from build123d import *

# Parameters (mm, degrees)
SKETCH1_R           = 6.22935
BOSS_EXTRUDE1_DEPTH = 31.75
SKETCH2_W           = 8.89
SKETCH2_H           = 31.75
CUT_EXTRUDE1_DEPTH  = 89.9


with BuildPart() as part:
    # Sketch1 → Boss-Extrude1 (new body)
    with BuildSketch(Plane(origin=(0, 0, 0), x_dir=(0, 0, -1), z_dir=(1, 0, 0))):
        with BuildLine():
            Line((22.594948, 7.845241626), (32.874076775, 30.623791868))
            ThreePointArc((32.874076775, 30.623791868), (44.45, 38.1), (56.025923225, 30.623791868))
            Line((56.025923225, 30.623791868), (66.305052, 7.845241626))
            ThreePointArc((66.305052, 7.845241626), (67.242210206, 6.756307629), (68.620236645, 6.35))
            Line((68.620236645, 6.35), (88.9, 6.35))
            Line((88.9, 6.35), (88.9, 0))
            Line((88.9, 0), (0, 0))
            Line((0, 0), (0, 6.35))
            Line((0, 6.35), (20.279763355, 6.35))
            ThreePointArc((20.279763355, 6.35), (21.657789794, 6.756307629), (22.594948, 7.845241626))
        make_face()
        with Locations((44.45, 25.4)):
            Circle(SKETCH1_R, mode=Mode.SUBTRACT)
    extrude(amount=-BOSS_EXTRUDE1_DEPTH)

    # Sketch2 → Cut-Extrude1 (cut, through all)
    with BuildSketch(Plane.XY):
        with Locations((-15.875, 22.225)):
            Rectangle(SKETCH2_W, SKETCH2_H)
    extrude(amount=-CUT_EXTRUDE1_DEPTH, mode=Mode.SUBTRACT)


solid = part.part
Can you work these out from the model? Positions are in its coordinate system, mm. A direction names the side the tool comes from. Give positions to 0.01 mm unless a question says otherwise; leave off trailing zeros. Loops run counter-clockwise (first coordinate to the right, second up) from the corner with the lowest first, then second, coordinate; pieces in that order, holes last. Notation, with made-up numbers: (30.5, 41) -> (67.5, 41) arc R12 ccw to (67.5, 53) -> close; hole circle Ø7 at (-6, -10.5). An arc over 180 degrees is marked (long way). Use one line per item in the form item = value.
1) I need wall thicknesses on line 1 along X through (y, z) = (9, -54); line 2 along Y through (x, z) = (-2.25, -44.45); line 3 along Y through (x, z) = (-14, -27). Which ranges of each line are inside material? Lowest first, please.
Answers:
line_1 = -31.75 to -20.32, -11.43 to 0
line_2 = 0 to 19.17, 31.63 to 38.1
line_3 = 0 to 6.35
2) If we section it at D-D (x = -15): Please give me the cut outline in (y, z), plus the area to 3 significant figures.
Answers:
outline = (0, -88.9) -> (6.35, -88.9) -> (6.35, 0) -> (0, 0) -> close
area = 565 mm²
3) We'd pull the mould along X, two halves only. Please class faces 1 (the face through (-11.43, 18, -44)), 2 (the face through (0, 15, -45)), 3 (the face through (-5.635, 6.745, -21.641)), 4 (the face through (-20.32, 18, -44)): released by +X, released by -X, zero draft, split by the parting line, or undercut.
Answers:
face_1 = undercut
face_2 = released by +X
face_3 = zero draft
face_4 = undercut
4) If we section it at A-A (z = -44.45): Please give me the cut outline in (x, y).
Answers:
outline = (-31.75, 0) -> (0, 0) -> (0, 19.17) -> (-11.43, 19.17) -> (-11.43, 6.35) -> (-20.32, 6.35) -> (-20.32, 19.17) -> (-31.75, 19.17) -> close; (-31.75, 31.63) -> (-20.32, 31.63) -> (-20.32, 38.1) -> (-31.75, 38.1) -> close; (-11.43, 31.63) -> (0, 31.63) -> (0, 38.1) -> (-11.43, 38.1) -> close
5) Will these pins go through, and if not, where does the flat tip stop? pin 1 (5 mm diameter, centred on x = -6.5, z = -50, fed in from +Y); pin 2 (5 mm diameter, centred on x = -27, y = 24.5, fed in from -Z); pin 3 (10 mm diameter, centred on x = -8.5, y = 32.5, fed in from -Z).
Answers:
pin_1 = 37.73
pin_2 = -59.92
pin_3 = -57.44
6) For faces 5 (the face through (-16, 6.35, -44)), 6 (the face through (-16, 3, 0)), which set-ups out of +Z, -Z, +X, -X, +Y, -Y let a thin tool reach every point of the face, with its end or its side?
Answers:
face_5 = +Y
face_6 = +Z, +X, -X, +Y, -Y
7) If we section it at B-B (y = 13): Please give me the cut outline in (x, z), plus the area to 3 significant figures.
Answers:
outline = (-31.75, -63.98) -> (-20.32, -63.98) -> (-20.32, -24.92) -> (-31.75, -24.92) -> close; (-11.43, -63.98) -> (0, -63.98) -> (0, -24.92) -> (-11.43, -24.92) -> close
area = 893 mm²
8) If we section it at C-C (y = 27.5): Please give me the cut outline in (x, z).
Answers:
outline = (-31.75, -57.44) -> (-20.32, -57.44) -> (-20.32, -50.31) -> (-31.75, -50.31) -> close; (-31.75, -38.59) -> (-20.32, -38.59) -> (-20.32, -31.46) -> (-31.75, -31.46) -> close; (-11.43, -57.44) -> (0, -57.44) -> (0, -50.31) -> (-11.43, -50.31) -> close; (-11.43, -38.59) -> (0, -38.59) -> (0, -31.46) -> (-11.43, -31.46) -> close
